Part model, mm, in its own coordinate system. A direction names the side the tool comes from. Give positions to 0.01 mm unless a question says otherwise; leave off trailing zeros. Order: outer loops, then holes, each group sorted by start corner. A loop starts at its lowest first (then second) coordinate and runs counter-clockwise, first axis right, second up. Notation, with made-up numbers: M -5.75,75.5 L 2.25,75.5 A22 ccw 2.25,110.5 Z; hole C -11.75,58.25 d4. An arc over 180 degrees is marked long. Answer as a JSON object with one key per item and string values.
from build123d import *

# Parameters (mm, degrees)
F0_R     = 1.5
F1_DEPTH = 10
F2_R     = 2.75
F3_DEPTH = 1.5
F5_DEPTH = 1.5


# Not quite as in the source:
# - a fillet or chamfer that OpenCascade refuses, or shapes differently, is made with other operations: its cross-section is extruded or revolved along the edge and cut away or added


with BuildPart() as f1:
    # F0 (on Front) → F1 (new body)
    with BuildSketch(Plane.XZ):
        Circle(F0_R)
    extrude(amount=F1_DEPTH)

    # F2 (on face) → F3 (join)
    with BuildSketch(Plane.XZ.offset(10)):
        Circle(F2_R)
    extrude(amount=F3_DEPTH)

    # F4 (on face) → F5 (cut)
    with BuildSketch(Plane.XZ.offset(11.5)):
        Polygon((-0.5773502692, -1), (0.5773502692, -1), (1.1547005384, 0), (0.5773502692, 1), (-0.5773502692, 1), (-1.1547005384, 0), align=None)
    extrude(amount=-F5_DEPTH, mode=Mode.SUBTRACT)

    # F6: fillet of radius 1.9 on 1 edges, made by hand

    # F6_s1 → F6_t2 (revolve, cut)
    with BuildSketch(Plane.XY):
        with BuildLine():
            ThreePointArc((2.75, -10), (2.0863160765, -11.0781745499), (0.8925824379, -11.5))
            Line((0.8925824379, -11.5), (2.75, -11.5))
            Line((2.75, -11.5), (2.75, -10))
        make_face()
    revolve(axis=Axis((0, -11.5, 0), (0, -1, 0)), mode=Mode.SUBTRACT)


solid = f1.part
1. Probe line 1 along Y through (x, z) = (0.15, 0.5); line 2 along Y through (x, z) = (-1.25, 0.65); line 3 along X through (y, z) = (-6, 1.15). List the from-to ranges inside material, lowest first.
Worked answers:
{"line 1": "y = -10 to 0", "line 2": "y = -11.43 to 0", "line 3": "x = -0.96 to 0.96"}
2. Two-plate mould, pull along Z, no slides. Class faces 3 (the flat face through (0.87, -10.76, 0.49)), 4 (the flat face through (0, 0, 0)), 5 (the cylindrical face through (-1.5, -4.93, 0.07)): +Z half, -Z half, draft (parallel to the pull), parting line (faces both ways), or undercut.
Worked answers:
{"face 3": "undercut", "face 4": "draft", "face 5": "parting line"}
3. Which spindle directions (+Z, -Z, +X, -X, +Y, -Y) get a long thin tool onto all of the face, cutting with end or side? Do faces 1 (the flat face through (1.2, -10, -1.2)), 2 (the flat face through (0.86, -10.76, -0.51)). Say none if no direction does.
Worked answers:
{"face 1": "+Y", "face 2": "-Y"}
4. Pin check, flat tips, straight feed: P1, Ø1.5, axis at x = 1.5, z = -2, coming from the -Y side; P2, Ø2, axis at x = 1, z = -1, coming from the -Y side; P3, Ø1, axis at y = -8.5, z = 1, coming from the +X side. Stop position of each tip, or through.
Worked answers:
{"P1": "stops at y = -11.3", "P2": "stops at y = -11.5", "P3": "stops at x = 1.41"}
5. Cut at A-A on y = -1.5. Give the cut face in (x, z), plus the area to 3 significant figures.
Worked answers:
{"outline": "C 0,0 d3", "area": "7.07 mm^2"}
